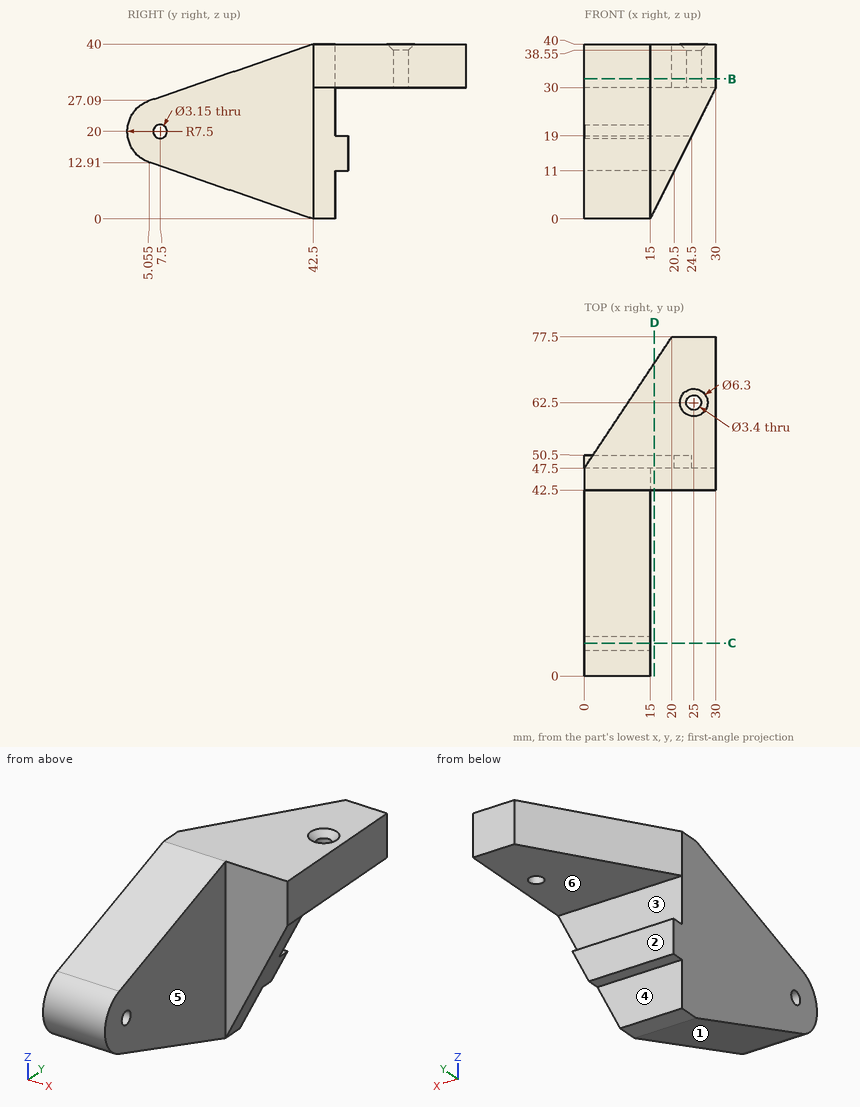
Part print with two shaded views. Sizes in mm from the minimum x, y, z corner. A direction names the side the tool comes from. Coordinates: 2 decimals unless noted, no trailing zeros. Loops run counter-clockwise (first coordinate to the right, second up) from the corner with the lowest first, then second, coordinate; pieces in that order, holes last. Notation, with made-up numbers: M 23,37 L 62,37 A17 ccw 62,63 Z; hole C 79.25,72.25 d11. An arc over 180 degrees is marked long. Use CSV: the item, a comma, the result in double quotes. Start each with the question number.
1. Two-plate mould, pull along Z, no slides. Class the marked faces 1, 2 and 3: pulls with the +Z half, pulls with the -Z half, needs draft (parallel to the pull), parting line crosses it, or undercut.
2. Band-saw the part on B-B, the plane z = 32. List the corners of the cut face in (x, y) (1 decimal), then the cut area to 3 significant figures.
3. Tool access for the marked faces 4, 5 and 6: list every direction of +Z, -Z, +X, -X, +Y, -Y with a clear straight run to the whole face (end or side of a thin tool).
4. Band-saw the part on D-D, the plane x = 16. List the corners of the cut face in (y, z).
5. Band-saw the part on C-C, the plane y = 7.5. List the corners of the cut face in (x, z) (1 decimal).
6. Flat gauge pins, fed straight in: pin 1 (3 mm diameter, centred on y = 11.5, z = 12.5, fed in from +X); pin 2 (6 mm diameter, centred on x = 11, z = 16, fed in from +Y); pin 3 (10 mm diameter, centred on y = 60, z = 21.5, fed in from +X); pin 4 (5.5 mm diameter, centred on x = 10.5, z = 22.5, fed in from +Y). Where does each tip first touch, or does it go through?
7. Probe probe 1 along Y at (x, z) = (25, 35); probe 2 along Y at (x, z) = (9.75, 20) (1 decimal); probe 3 along X at (y, z) = (22.5, 8). List the from-to ranges inside material, lowest first. Write a range as [from, to].
Entries:
1,face 1,"pulls with the -Z half"
1,face 2,"needs draft"
1,face 3,"undercut"
2,outline,"M 0,19.3 L 15,19.3 L 15,42.5 L 30,42.5 L 30,77.5 L 20,77.5 L 0,47.5 Z; hole C 25,62.5 d3.4"
2,area,"1,090 mm2"
3,face 4,"-Z, +X, -X, +Y"
3,face 5,"+Z, -Z, +X, -Y"
3,face 6,"+X, -X, +Y"
4,outline,"M 42.5,2 L 47.5,2 L 47.5,11 L 50.5,11 L 50.5,19 L 47.5,19 L 47.5,30 L 71.5,30 L 71.5,40 L 42.5,40 Z"
5,outline,"M 0,12.1 L 15,12.1 L 15,18.4 L 0,18.4 Z; M 0,21.6 L 15,21.6 L 15,27.9 L 0,27.9 Z"
6,pin 1,"stops at x = 15"
6,pin 2,"stops at y = 50.5"
6,pin 3,"passes through"
6,pin 4,"stops at y = 47.5"
7,probe 1,"y = [42.5, 60.8], [64.2, 77.5]"
7,probe 2,"y = [0, 5.9], [9.1, 47.5]"
7,probe 3,"x = [0, 15]"
